Read the model definition and answer for the solid it produces. Units are mm, in the model's axes. Give positions to 0.01 mm unless a question says otherwise; leave off trailing zeros. Order: outer loops, then holes, each group sorted by start corner. A loop starts at its lowest first (then second) coordinate and runs counter-clockwise, first axis right, second up.
Item 1: A cutting plane is placed at A-A (z = -20). Write down the section's boundary in (x, y), plus the area to 3 significant figures.
Item 2: Given pin 1 Ø1.8 at (x, z) = (-19, 4) entering from +Y; pin 2 Ø3.5 at (x, z) = (-4, -20) entering from +Y, each flat-ended and moving along its own axis, determine where each tip first touches the part or whether it passes through.
Item 3: A cutting plane is placed at B-B (y = -4.3). Write down the section's boundary in (x, z).
Item 4: Find the intervals of material crossed by line 1 along Z through (x, y) = (-5, -1.7); line 2 along Z through (x, y) = (-3, -3.4); line 3 along Z through (x, y) = (-18.25, -3.8), in increasing order.
Item 5: A cutting plane is placed at C-C (x = -6.5). Write down the section's boundary in (y, z).
Item 6: A cutting plane is placed at D-D (z = -2). Write down the section's boundary in (x, y).
Autodesk Inventor part; units mm, degrees
ref_plane "YZ Plane" through (0, 0, 0) normal (1, 0, 0) x (0, 1, 0)
ref_plane "XZ Plane" through (0, 0, 0) normal (0, 1, 0) x (-1, 0, 0)
ref_plane "XY Plane" through (0, 0, 0) normal (0, 0, 1) x (1, 0, 0)
sketch "스케치1" plane through (0, 0, 0) normal (0, 1, 0) x (-1, 0, 0)
  line L0 (0, 0) -> (24, 0)
  line L1 (24, 0) -> (24, -24)
  line L2 (24, -24) -> (0, -24)
  line L3 (0, -24) -> (0, 0)
  circle A0 centre (4, -4) radius 1.1
  circle A1 centre (4, -4) radius 2.1
  line L4 (1.9, -4) -> (4, -4)
  line L5 (1.9, -2.7876) -> (4, -1.5751)
  line L6 (4, -1.5751) -> (6.1, -2.7876)
  line L7 (6.1, -2.7876) -> (6.1, -5.2124)
  line L8 (6.1, -5.2124) -> (4, -6.4249)
  line L9 (4, -6.4249) -> (1.9, -5.2124)
  line L10 (1.9, -5.2124) -> (1.9, -2.7876)
  circle A2 centre (4, -20) radius 1.1
  circle A3 centre (4, -20) radius 2.1
  line L11 (1.9, -20) -> (4, -20)
  line L12 (1.9, -18.7876) -> (4, -17.5751)
  line L13 (4, -17.5751) -> (6.1, -18.7876)
  line L14 (6.1, -18.7876) -> (6.1, -21.2124)
  line L15 (6.1, -21.2124) -> (4, -22.4249)
  line L16 (4, -22.4249) -> (1.9, -21.2124)
  line L17 (1.9, -21.2124) -> (1.9, -18.7876)
  circle A4 centre (20, -4) radius 1.1
  circle A5 centre (20, -4) radius 2.1
  line L18 (17.9, -4) -> (20, -4)
  line L19 (17.9, -2.7876) -> (20, -1.5751)
  line L20 (20, -1.5751) -> (22.1, -2.7876)
  line L21 (22.1, -2.7876) -> (22.1, -5.2124)
  line L22 (22.1, -5.2124) -> (20, -6.4249)
  line L23 (20, -6.4249) -> (17.9, -5.2124)
  line L24 (17.9, -5.2124) -> (17.9, -2.7876)
  circle A6 centre (20, -20) radius 1.1
  circle A7 centre (20, -20) radius 2.1
  line L25 (17.9, -20) -> (20, -20)
  line L26 (17.9, -18.7876) -> (20, -17.5751)
  line L27 (20, -17.5751) -> (22.1, -18.7876)
  line L28 (22.1, -18.7876) -> (22.1, -21.2124)
  line L29 (22.1, -21.2124) -> (20, -22.4249)
  line L30 (20, -22.4249) -> (17.9, -21.2124)
  line L31 (17.9, -21.2124) -> (17.9, -18.7876)
  line L32 (12, 0) -> (12, 4)
  line L33 (12, 4) -> (19, 4)
  line L34 (12, 4) -> (5, 4)
  dimension "d3" = 4.2
  dimension "d0" = 24
  dimension "d1" = 24
  dimension "d2" = 2.2
  dimension "d6" = 16
  dimension "d9" = 16
  dimension "d12" = 4
  dimension "d13" = 7
  dimension "d14" = 7
extrude "돌출1" add sketch "스케치1" against normal blind 5 contours L0 L1 L2 L3 | A0 | A1 | A1 L9 L10 | L10 L5 A1 | L5 L6 A1 | A1 L8 L9 | L6 L7 A1 | A1 L7 L8 | A2 | A3 | A3 L16 L17 | L17 L12 A3 | L12 L13 A3 | A3 L15 L16 | L13 L14 A3 | A3 L14 L15 | A4 | A5 | A5 L23 L24 | L24 L19 A5 | L19 L20 A5 | A5 L22 L23 | L20 L21 A5 | A5 L21 L22 | A6 | A7 | A7 L30 L31 | L31 L26 A7 | L26 L27 A7 | A7 L29 L30 | L27 L28 A7 | A7 L28 L29
extrude "돌출2" cut sketch "스케치1" against normal blind 2 contours A0 | A1 | A1 L9 L10 | L10 L5 A1 | L5 L6 A1 | A1 L8 L9 | L6 L7 A1 | A1 L7 L8 | A2 | A3 | A3 L16 L17 | L17 L12 A3 | L12 L13 A3 | A3 L15 L16 | L13 L14 A3 | A3 L14 L15 | A4 | A5 | A5 L23 L24 | L24 L19 A5 | L19 L20 A5 | A5 L22 L23 | L20 L21 A5 | A5 L21 L22 | A6 | A7 | A7 L30 L31 | L31 L26 A7 | L26 L27 A7 | A7 L29 L30 | L27 L28 A7 | A7 L28 L29
extrude "돌출3" cut sketch "스케치1" against normal blind 5 contours A0 | A2 | A4 | A6
sketch "스케치2" plane through (0, 0, 0) normal (0, 1, 0) x (1, 0, 0)
  line L0 (0, 0) -> (-24, 0)
  line L1 (-24, 0) -> (-24, -8)
  line L2 (-24, -8) -> (0, -8)
  line L3 (0, -8) -> (0, 0)
  dimension "d21" = 8
extrude "돌출4" add sketch "스케치2" against normal blind 5
sketch "스케치3" plane through (0, -5, 0) normal (0, -1, 0) x (1, 0, 0)
  line L0 (0, 0) -> (-12, 0)
  line L1 (-12, 0) -> (-12, 4)
  line L2 (-12, 4) -> (-5, 4)
  line L3 (-12, 4) -> (-19, 4)
  circle A0 centre (-5, 4) radius 1.1
  circle A1 centre (-5, 4) radius 2.1
  circle A2 centre (-19, 4) radius 1.1
  circle A3 centre (-19, 4) radius 2.1
  line L4 (-2.9, 2.7876) -> (-5, 1.5751)
  line L5 (-5, 1.5751) -> (-7.1, 2.7876)
  line L6 (-7.1, 2.7876) -> (-7.1, 5.2124)
  line L7 (-7.1, 5.2124) -> (-5, 6.4249)
  line L8 (-5, 6.4249) -> (-2.9, 5.2124)
  line L9 (-2.9, 5.2124) -> (-2.9, 2.7876)
  line L10 (-21.1, 5.2124) -> (-19, 6.4249)
  line L11 (-19, 6.4249) -> (-16.9, 5.2124)
  line L12 (-16.9, 5.2124) -> (-16.9, 2.7876)
  line L13 (-16.9, 2.7876) -> (-19, 1.5751)
  line L14 (-19, 1.5751) -> (-21.1, 2.7876)
  line L15 (-21.1, 2.7876) -> (-21.1, 5.2124)
  point P0 (-2.9, 4)
  point P1 (-21.1, 4)
  dimension "d29" = 4.2
  dimension "d31" = 4.2
  dimension "d24" = 12
  dimension "d25" = 4
  dimension "d26" = 7
  dimension "d27" = 7
  dimension "d28" = 2.2
  dimension "d30" = 2.2
extrude "돌출5" cut sketch "스케치3" against normal blind 2 contours L6 L7 A1 | A0 | A1 | A1 L5 L6 | L12 L13 A3 | A2 | A3 | A3 L11 L12 | L7 L8 A1 | A1 L4 L5 | A3 L10 L11 | L13 L14 A3 | L8 L9 A1 | A1 L9 L4 | A3 L15 L10 | L14 L15 A3
extrude "돌출6" cut sketch "스케치3" against normal blind 5 contours A0 | A2
properties part number "robot_left"
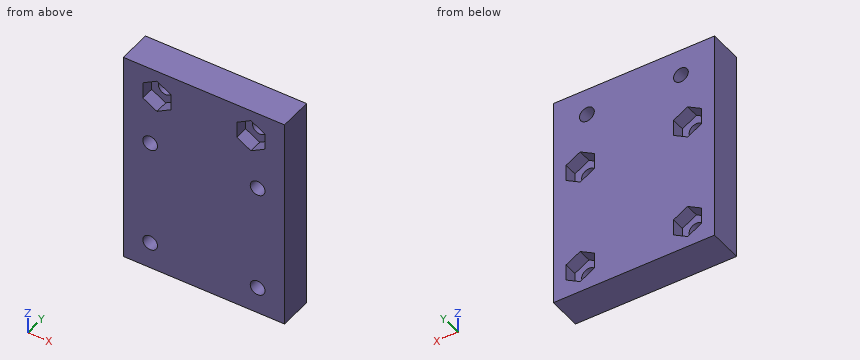
Response values:
1. outline: (-24, -5) - (-21.1, -5) - (-21.1, -2) - (-22.1, -2) - (-22.1, 0) - (-24, 0) - close; (-18.9, -5) - (-5.1, -5) - (-5.1, -2) - (-6.1, -2) - (-6.1, 0) - (-17.9, 0) - (-17.9, -2) - (-18.9, -2) - close; (-2.9, -5) - (0, -5) - (0, 0) - (-1.9, 0) - (-1.9, -2) - (-2.9, -2) - close
1. area: 90.0 mm2
2. pin 1: passes through
2. pin 2: stops at y = -2
3. outline: (-24, -24) - (0, -24) - (0, 8) - (-24, 8) - close; hole circle Ø2.2 at (-20, -20); hole circle Ø2.2 at (-20, -4); hole (-21.1, 2.79) - (-19, 1.58) - (-16.9, 2.79) - (-16.9, 5.21) - (-19, 6.42) - (-21.1, 5.21) - close; hole (-7.1, 2.79) - (-5, 1.58) - (-2.9, 2.79) - (-2.9, 5.21) - (-5, 6.42) - (-7.1, 5.21) - close; hole circle Ø2.2 at (-4, -20); hole circle Ø2.2 at (-4, -4)
4. line 1: z = -24 to -21.85, -18.15 to -5.85, -2.15 to 2.9, 5.1 to 8
4. line 2: z = -24 to -20.46, -19.54 to -4.46, -3.54 to 2.73, 5.27 to 8
4. line 3: z = -24 to 2.01, 5.99 to 8
5. outline: (-5, -24) - (0, -24) - (0, 8) - (-5, 8) - (-5, 5.56) - (-3, 5.56) - (-3, 2.44) - (-5, 2.44) - close
6. outline: (-24, -5) - (0, -5) - (0, 0) - (-3.26, 0) - (-3.26, -2) - (-4.74, -2) - (-4.74, 0) - (-19.26, 0) - (-19.26, -2) - (-20.74, -2) - (-20.74, 0) - (-24, 0) - close
